Verification items for this drawing (mm, ordinates from the low corner). A direction names the side the tool comes from. Round coordinates to 2 decimals unless told otherwise and drop trailing zeros. Write each loop counter-clockwise with the first axis right and the second up, starting at its lowest first coordinate (ties: lowest second). Pieces come first, ordered by that corner, then holes.
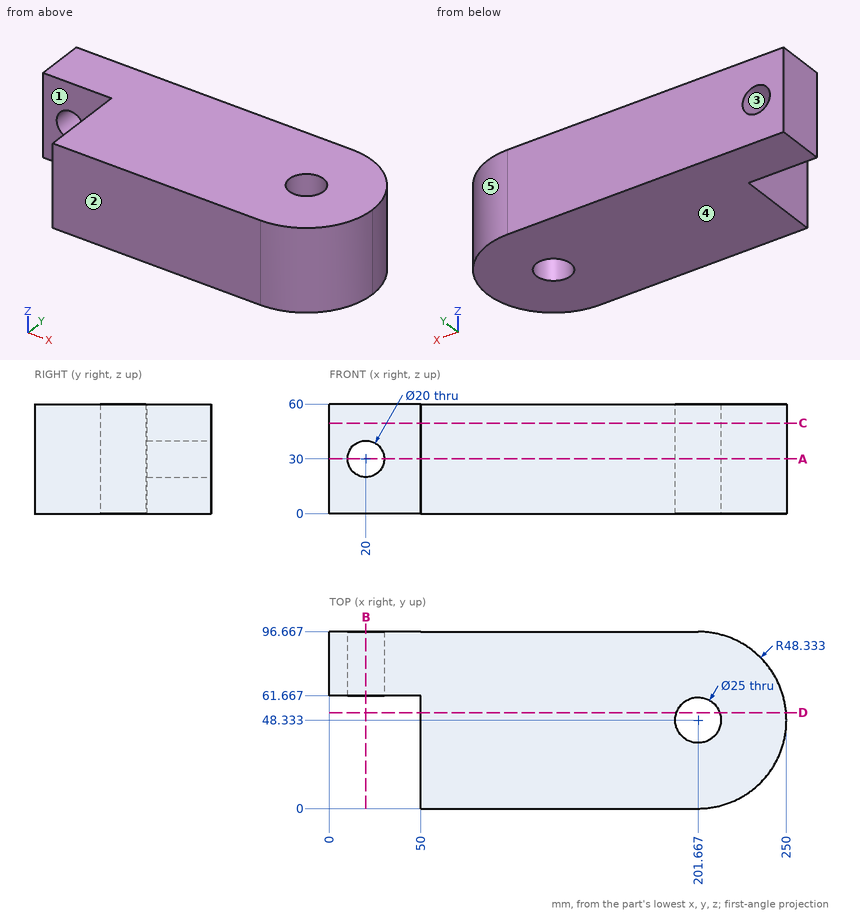
1. Section check A-A (z = 30). Record the cut outline in (x, y).
2. Section check B-B (x = 20). Record the cut outline in (y, z).
3. Release check for a two-part mould opening along X. For the marked faces 3, 4 and 5 record: +X half, -X half, draft (parallel to the pull), parting line (faces both ways), or undercut.
4. Depth check by flat-ended pin: pin 1 Ø4 at (x, y) = (210.5, 42.5) entering from -Z; pin 2 Ø5 at (y, z) = (13.5, 29) entering from +X; pin 3 Ø10 at (y, z) = (65, 15) entering from +X. Enter the tip coordinate at first touch or a pass-through.
5. Scan lines: line 1 along Z through (x, y) = (20, 70.5); line 2 along Y through (x, z) = (35, 52); line 3 along X through (y, z) = (88, 30) (1 decimal). Record each from-to range of solid material in increasing order.
6. Section check D-D (y = 52.5). Record the cut outline in (x, z), plus the area to 3 significant figures.
7. Access from +Z, -Z, +X, -X, +Y, -Y to the whole of each face (thin tool, end or side, straight path). Record for the marked faces 1 and 2.
8. Section check C-C (z = 49.5). Record the cut outline in (x, y), plus the area to 3 significant figures.
Results below:
1. outline: (0, 61.67) - (10, 61.67) - (10, 96.67) - (0, 96.67) - close; (30, 61.67) - (50, 61.67) - (50, 0) - (201.67, 0) arc R48.33 ccw to (201.67, 96.67) - (30, 96.67) - close; hole circle Ø25 at (201.67, 48.33)
2. outline: (61.67, 0) - (96.67, 0) - (96.67, 20) - (61.67, 20) - close; (61.67, 40) - (96.67, 40) - (96.67, 60) - (61.67, 60) - close
3. face 3: undercut
3. face 4: draft
3. face 5: +X half
4. pin 1: stops at z = 0
4. pin 2: stops at x = 237.59
4. pin 3: stops at x = 248.57
5. line 1: z = 0 to 20, 40 to 60
5. line 2: y = 61.67 to 96.67
5. line 3: x = 0 to 10, 30 to 229.3
6. outline: (50, 0) - (189.88, 0) - (189.88, 60) - (50, 60) - close; (213.45, 0) - (249.82, 0) - (249.82, 60) - (213.45, 60) - close
6. area: 10,600 mm2
7. face 1: +Z, -Z, -X, -Y
7. face 2: +Z, -Z, +X, -X, -Y
8. outline: (0, 61.67) - (50, 61.67) - (50, 0) - (201.67, 0) arc R48.33 ccw to (201.67, 96.67) - (0, 96.67) - close; hole circle Ø25 at (201.67, 48.33)
8. area: 19,600 mm2
